```python
from build123d import *

# Parameters (mm, degrees)
CHAMFER_SIZE = 0.2


with BuildPart() as part:
    # Sketch → Revolution (revolve)
    with BuildSketch(Plane.XY):
        with BuildLine():
            Line((3, 6.6), (3, 9.5))
            Line((2.1, 9.5), (3, 9.5))
            ThreePointArc((-2.1, 9.5), (0, 7.4), (2.1, 9.5))
            Line((-3, 9.5), (-2.1, 9.5))
            Line((-3, 9.5), (-3, 6.6))
            Line((-3, 6.6), (3, 6.6))
        make_face()
    revolve(axis=Axis((0, 0, 0), (1, 0, 0)))

    # Chamfer
    chamfer_edges = [part.edges().sort_by_distance(p)[0] for p in [
        (-3, -6.6, 0),
        (-3, -9.5, 0),
        (3, -9.5, 0),
        (3, -6.6, 0),
    ]]
    chamfer(chamfer_edges, length=CHAMFER_SIZE)


solid = part.part
```
Input: part model. Units: mm. Frame: model coordinates. Give positions to 0.01 mm unless a question says otherwise; leave off trailing zeros. Loops run counter-clockwise (first coordinate to the right, second up) from the corner with the lowest first, then second, coordinate; pieces in that order, holes last. Notation, with made-up numbers: M 12.25,74.5 L 23.25,74.5 A24 ccw 23.25,111.5 Z; hole C -6.5,22.25 d10. An arc over 180 degrees is marked long. Answer as CSV lines item,"result". Start each with the question number.
1. Section A-A on y = 0. Return loops of the section in (x, z), plus the area to 3 significant figures.
2. Pull-direction query (Y, two-part tool) for faces 1 (the face through (0.039, -4.864, 4.461)), 2 (the face through (-2.45, 4.38, -8.43)), 3 (the face through (3, -1, -7)); classes: released by +Y, released by -Y, zero draft, split by the parting line, or undercut.
3. Pin query (flat end, axial travel): P1, Ø1.5, axis at y = 3, z = -4.5, coming from the +X side; P2, Ø6, axis at y = 4.5, z = -4, coming from the -X side. Return the tip coordinate at first contact, or that it passes through.
4. Section D-D on x = -1.6. Return loops of the section in (y, z), plus the area to 3 significant figures.
5. Line query: L1, parallel to X at y = 7.25, z = -5.5; L2, parallel to Z at x = -1.6, y = 0; L3, parallel to X at y = -2.5, z = -7.25. Output: solid intervals per line, ascending.
6. Section C-C on x = -0.3. Return loops of the section in (y, z).
Computed values:
1,outline,"M -3,-9.3 L -2.8,-9.5 L -2.1,-9.5 A2.1 cw 2.1,-9.5 L 2.8,-9.5 L 3,-9.3 L 3,-6.8 L 2.8,-6.6 L -2.8,-6.6 L -3,-6.8 Z; M -3,6.8 L -2.8,6.6 L 2.8,6.6 L 3,6.8 L 3,9.3 L 2.8,9.5 L 2.1,9.5 A2.1 cw -2.1,9.5 L -2.8,9.5 L -3,9.3 Z"
1,area,"20.8 mm²"
2,face 1,"undercut"
2,face 2,"split by the parting line"
2,face 3,"zero draft"
3,P1,"passes through"
3,P2,"stops at x = -3"
4,outline,"C 0,0 d16.28; hole C 0,0 d13.2"
4,area,"71.3 mm²"
5,L1,"x = -3 to -2.06, 2.06 to 3"
5,L2,"z = -8.14 to -6.6, 6.6 to 8.14"
5,L3,"x = -3 to -1.03, 1.03 to 3"
6,outline,"C 0,0 d14.84; hole C 0,0 d13.2"
